Geometry check sheet. Reference: drawing and pictorial views, mm from the part's lowest x, y, z. A direction names the side the tool comes from. Give positions to 0.01 mm unless a question says otherwise; leave off trailing zeros. Loops run counter-clockwise (first coordinate to the right, second up) from the corner with the lowest first, then second, coordinate; pieces in that order, holes last. Notation, with made-up numbers: (17.5, 29) -> (41.5, 29) arc R7 cw to (41.5, 39) -> close; hole circle Ø7 at (-14.5, 25.5). An arc over 180 degrees is marked (long way). One line per item, written item: value. Start each with the question number.
(1) Sectioned sample at C-C, the plane y = 0.5. Record the cut outline in (x, z), then the cut area to 3 significant figures.
(2) Sectioned sample at D-D, the plane y = 4. Record the cut outline in (x, z), then the cut area to 3 significant figures.
(3) Sectioned sample at B-B, the plane x = 12. Record the cut outline in (y, z).
(4) Sectioned sample at A-A, the plane z = 8. Record the cut outline in (x, y), then the cut area to 3 significant figures.
(5) Scan lines: line 1 along X through (y, z) = (5, 1.65); line 2 along X through (y, z) = (1, 8); line 3 along Y through (x, z) = (3.5, 4). Record each from-to range of solid material in increasing order. Write a range as from..to.
(6) Tool access check on the marked faces 1 and 2. Record the directions out of +Z, -Z, +X, -X, +Y, -Y that give a thin tool (end or side, any length) a straight path to the whole face; none if there is none.
(7) Gauge pin test, flat ends, axial feed: pin 1 Ø2 at (x, z) = (41, 6.5) entering from +Y; pin 2 Ø4 at (y, z) = (8, 5) entering from +X; pin 3 Ø1 at (x, y) = (44, 5) entering from +Z. Record the tip position at first contact, or that the pin passes through.
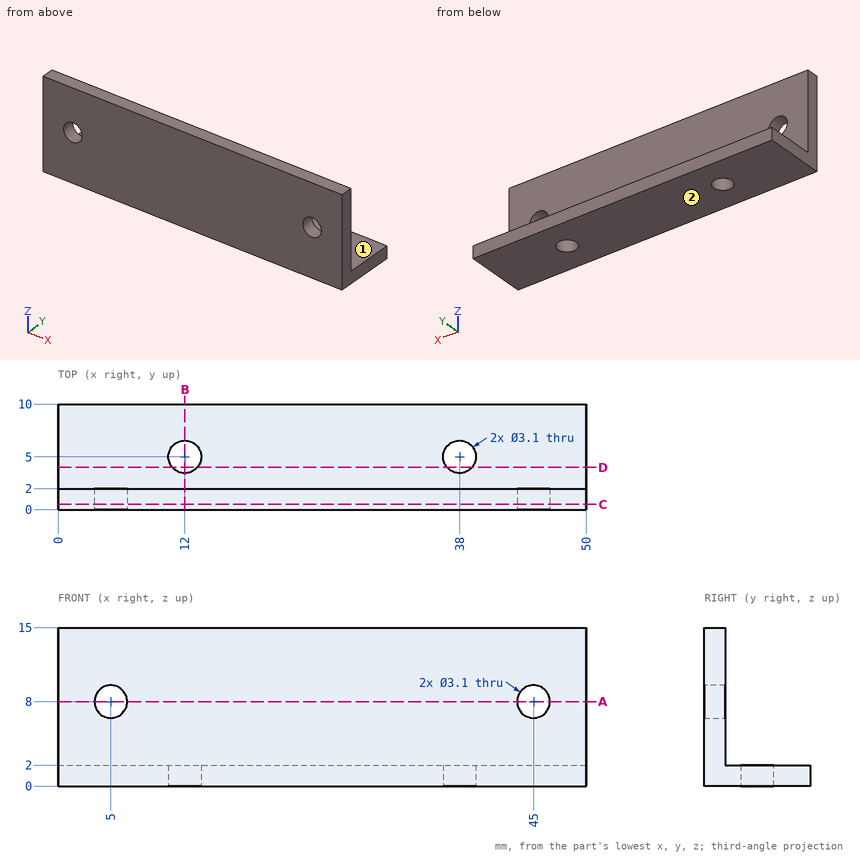
Calculated:
1. outline: (0, 0) -> (50, 0) -> (50, 15) -> (0, 15) -> close; hole circle Ø3.1 at (5, 8); hole circle Ø3.1 at (45, 8)
1. area: 735 mm2
2. outline: (0, 0) -> (10.82, 0) -> (10.82, 2) -> (0, 2) -> close; (13.18, 0) -> (36.82, 0) -> (36.82, 2) -> (13.18, 2) -> close; (39.18, 0) -> (50, 0) -> (50, 2) -> (39.18, 2) -> close
2. area: 90.5 mm2
3. outline: (0, 0) -> (3.45, 0) -> (3.45, 2) -> (2, 2) -> (2, 15) -> (0, 15) -> close; (6.55, 0) -> (10, 0) -> (10, 2) -> (6.55, 2) -> close
4. outline: (0, 0) -> (3.45, 0) -> (3.45, 2) -> (0, 2) -> close; (6.55, 0) -> (43.45, 0) -> (43.45, 2) -> (6.55, 2) -> close; (46.55, 0) -> (50, 0) -> (50, 2) -> (46.55, 2) -> close
4. area: 87.6 mm2
5. line 1: x = 0..10.45, 13.55..36.45, 39.55..50
5. line 2: x = 0..3.45, 6.55..43.45, 46.55..50
5. line 3: y = 0..2
6. face 1: +Z, +X, -X, +Y
6. face 2: -Z, +X, -X, +Y, -Y
7. pin 1: stops at y = 2
7. pin 2: passes through
7. pin 3: stops at z = 2
